Autodesk Inventor part; units mm, degrees
ref_plane "Work Plane1" through (-22.1363, -57.0374, 30) normal (0, 0, 1) x (1, 0, 0)
ref_plane "Work Plane4" through (-22.1363, -57.0374, 0) normal (0, -1, 0) x (1, 0, 0)
ref_plane "YZ Plane" through (0, 0, 0) normal (1, 0, 0) x (0, 1, 0)
ref_plane "Work Plane1" through (-22.1363, -57.0374, 30) normal (0, 0, 1) x (1, 0, 0)
sketch "Sketch1" plane through (-22.1363, -57.0374, 30) normal (0, 0, 1) x (1, 0, 0)
  line L0 (0, 0) -> (50, 0)
  line L1 (50, 0) -> (50, 81)
  line L2 (50, 81) -> (0, 81)
  line L3 (0, 81) -> (0, 0)
  line L4 (25, 81) -> (25, 0) construction
  line L5 (0, 40.5) -> (50, 40.5) construction
  circle A0 centre (5, 76) radius 2.25
  circle A1 centre (45, 5) radius 2.25
  circle A2 centre (45, 76) radius 2.25
  circle A3 centre (5, 5) radius 2.25
  line L6 (18, 81) -> (18, 0)
  line L7 (32, 81) -> (32, 0)
  line L8 (0, 15) -> (50, 15)
  line L9 (0, 57) -> (50, 57)
  circle A4 centre (35, 30.5) radius 1.6
  circle A5 centre (15, 50.5) radius 1.6
  circle A6 centre (15, 30.5) radius 1.6
  circle A7 centre (35, 50.5) radius 1.6
  point P0 (18, 57)
  point P1 (32, 57)
  dimension "d0" = 50
  dimension "d1" = 81
  dimension "d2" = 5
  dimension "d3" = 5
  dimension "d5" = 4.5
  dimension "d27" = 14
  dimension "d28" = 24
  dimension "d29" = 15
  dimension "d30" = 20
  dimension "d31" = 20
  dimension "d32" = 3.2
ref_plane "Work Plane4" through (-22.1363, -57.0374, 0) normal (0, -1, 0) x (1, 0, 0)
sketch "Sketch2" plane through (-22.1363, -57.0374, 0) normal (0, -1, 0) x (1, 0, 0)
  line L0 (0, 0) -> (50, 0)
  line L1 (50, 0) -> (50, 30)
  line L2 (50, 30) -> (0, 30)
  line L3 (0, 30) -> (0, 0)
  line L4 (25, 0) -> (25, 30) construction
  line L5 (0, 12) -> (50, 12) construction
  circle A0 centre (25, 12) radius 5.1
  circle A1 centre (30.6569, 17.6569) radius 2.25
  line L6 (25, 12) -> (30.6569, 17.6569) construction
  circle A2 centre (19.3431, 6.3431) radius 2.25
  circle A3 centre (30.6569, 6.3431) radius 2.25
  circle A4 centre (19.3431, 17.6569) radius 2.25
  dimension "d17" = 50
  dimension "d18" = 30
  dimension "d21" = 12
  dimension "d22" = 10.2
  dimension "d24" = 4.5
  dimension "d25" = 8
  dimension "d26" = 45
extrude "Extrusion1" add sketch "Sketch1" against normal blind 30 contours L3 L8 L6 L0 | L6 L8 L7 L0 | L3 L9 L6 L8 | L7 L8 L1 L0 | L6 L9 L7 L8 | L3 L2 L6 L9 | L7 L9 L1 L8 | L6 L2 L7 L9 | L7 L2 L1 L9 | A0 | A1 | A2 | A3 | A4 | A5 | A6 | A7
hole "Hole2" at (-7.1363, -6.5374, 30) at (12.8637, -6.5374, 30) at (12.8637, -26.5374, 30) at (-7.1363, -26.5374, 30) direction (0, 0, -1) diameter 3.2 end through all
hole "Hole3" at (-17.1363, 18.9626, 30) at (22.8637, 18.9626, 30) at (22.8637, -52.0374, 30) at (-17.1363, -52.0374, 30) direction (0, 0, -1) diameter 4.5 end through all
hole "Hole4" at (-2.7932, -57.0374, 17.6569) at (8.5205, -57.0374, 17.6569) at (8.5205, -57.0374, 6.3431) at (-2.7932, -57.0374, 6.3431) direction (0, 1, 0) diameter 4.5 depth 15
hole "Hole5" at (2.8637, -57.0374, 12) direction (0, 1, 0) diameter 10.2 end through all
extrude "Extrusion2" cut sketch "Sketch1" against normal blind 25 contours L3 L9 L6 L8 | L6 L9 L7 L8 | L7 L9 L1 L8 | L6 L2 L7 L9
properties part number "y_slider_bracket" material "PC/ABS Plastic"
Geometry: final body of the model. Coordinates: model frame, mm. A direction names the side the tool comes from. Round coordinates to 2 decimals unless told otherwise and drop trailing zeros. Loops run counter-clockwise (first coordinate to the right, second up) from the corner with the lowest first, then second, coordinate; pieces in that order, holes last. Notation, with made-up numbers: M 6,22.5 L 27,22.5 A31 ccw 27,46.5 Z; hole C 35,72 d2. An arc over 180 degrees is marked long. Put each result on its own line as item: value. Start each with the question number.
(1) Draft query along Y for faces 5 (the face through (7, -49.432, 19.315)), 6 (the face through (3, -57.037, 19)), 7 (the face through (-18.66, 20.62, 14.79)), 8 (the face through (14, 23.963, 15)). Return one class per face: +Y half, -Y half, draft (parallel to the pull), parting line (faces both ways), or undercut.
(2) Section query A-A (z = 12). Return loops of the section in (x, y).
(3) Contact query for a flat-ended pin moving along its axis: pin 1 Ø3.5 at (x, y) = (-17.14, 18.96) entering from -Z. Output: stop coordinate, or through.
(4) Section query D-D (z = 2.5). State how many separate pieces and enclosed holes the cut face has, then the cut area to 3 significant figures.
(5) Section query B-B (y = 6). Return loops of the section in (x, z), then the cut area to 3 significant figures.
(6) Section query C-C (y = -45). Return loops of the section in (x, z), then the cut area to 3 significant figures.
(7) Set-up query: faces 1 (the face through (3, -49, 30)), 2 (the face through (-2.892, -49.432, 19.905)), 3 (the face through (19, -0.037, 18)), 4 (the face through (9.864, 12, 18)). Return all of +Z, -Z, +X, -X, +Y, -Y with unobstructed straight access to the full face (end or side cutting, diameter ignored); none if empty.
(8) Material intervals for line 1 along Y through (x, z) = (-8, 23.75); line 2 along X through (y, z) = (3, 28.75); line 3 along X through (y, z) = (17, 15.25), sorted ascending. Write a range as [from, to].
Findings below:
1. face 5: draft
1. face 6: -Y half
1. face 7: undercut
1. face 8: +Y half
2. outline: M -22.14,-57.04 L -2.24,-57.04 L -2.24,-42.04 L -22.14,-42.04 Z; M -22.14,-0.04 L -4.14,-0.04 L -4.14,23.96 L -22.14,23.96 Z; M 7.96,-57.04 L 27.86,-57.04 L 27.86,-42.04 L 7.96,-42.04 Z; M 9.86,-0.04 L 27.86,-0.04 L 27.86,23.96 L 9.86,23.96 Z; hole C -17.14,-52.04 d4.5; hole C -17.14,18.96 d4.5; hole C 22.86,-52.04 d4.5; hole C 22.86,18.96 d4.5
3. pin 1: passes through
4. separate pieces: 1
4. enclosed holes: 8
4. area: 3,950 mm2
5. outline: M -22.14,0 L 27.86,0 L 27.86,30 L 9.86,30 L 9.86,5 L -4.14,5 L -4.14,30 L -22.14,30 Z
5. area: 1,150 mm2
6. outline: M -22.14,0 L 27.86,0 L 27.86,30 L -22.14,30 Z; hole C -2.79,6.34 d4.5; hole C -2.79,17.66 d4.5; hole C 2.86,12 d10.2; hole C 8.52,6.34 d4.5; hole C 8.52,17.66 d4.5
6. area: 1,350 mm2
7. face 1: +Z, +X, -X, +Y, -Y
7. face 2: -Y
7. face 3: +Z, +X, -X
7. face 4: +Z, +Y
8. line 1: y = [-57.04, -42.04], [-0.04, 23.96]
8. line 2: x = [-22.14, -4.14], [9.86, 27.86]
8. line 3: x = [-22.14, -18.24], [-16.04, -4.14], [9.86, 21.76], [23.96, 27.86]
